Print and shaded views of the part. All mm, measured from the part's lowest x, y and z. A direction names the side the tool comes from. Round coordinates to 2 decimals unless told otherwise and drop trailing zeros. Write each loop counter-clockwise with the first axis right and the second up, starting at its lowest first coordinate (ties: lowest second). Pieces come first, ordered by that corner, then holes.
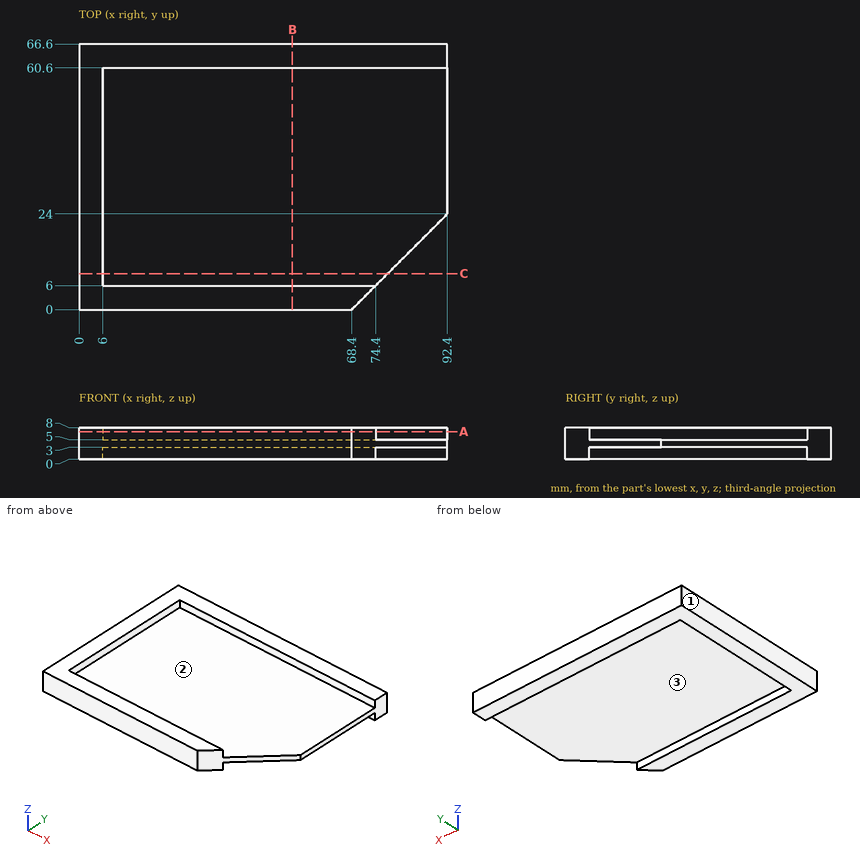
1) Wall check: L1, parallel to Y at x = 65.5, z = 2.75; L2, parallel to Z at x = 48.5, y = 7.5; L3, parallel to X at y = 31, z = 2.75. Give the ranges that are in metal, low to high.
Results:
L1: y = 0 to 6, 60.6 to 66.6
L2: z = 3 to 5
L3: x = 0 to 6
2) Slice it at A-A (z = 7). Write the cut outline in (x, y), plus the area to 3 significant figures.
Results:
outline: (0, 0) - (68.4, 0) - (74.4, 6) - (6, 6) - (6, 60.6) - (92.4, 60.6) - (92.4, 66.6) - (0, 66.6) - close
area: 1,310 mm2
3) Slice it at C-C (y = 9). Write the cut outline in (x, z).
Results:
outline: (0, 0) - (6, 0) - (6, 3) - (77.4, 3) - (77.4, 5) - (6, 5) - (6, 8) - (0, 8) - close
4) Pin check, flat tips, straight feed: pin 1 Ø4 at (x, z) = (80.5, 2.5) entering from -Y; pin 2 Ø1 at (x, y) = (36, 17.5) entering from -Z; pin 3 Ø1.5 at (y, z) = (25.5, 1.5) entering from +X; pin 4 Ø1.5 at (x, y) = (79, 9) entering from +Z. Stop position of each tip, or through.
Results:
pin 1: stops at y = 10.16
pin 2: stops at z = 3
pin 3: stops at x = 6
pin 4: passes through
5) Which spindle directions (+Z, -Z, +X, -X, +Y, -Y) get a long thin tool onto all of the face, cutting with end or side? Do the marked faces 1, 2 and 3. Say none if no direction does.
Results:
face 1: +Z, -Z, -X, +Y, -Y
face 2: +Z, +X
face 3: -Z, +X
6) Slice it at B-B (x = 53.5). Write the cut outline in (y, z).
Results:
outline: (0, 0) - (6, 0) - (6, 3) - (60.6, 3) - (60.6, 0) - (66.6, 0) - (66.6, 8) - (60.6, 8) - (60.6, 5) - (6, 5) - (6, 8) - (0, 8) - close
